Input: part model. Units: mm. Frame: model coordinates. A direction names the side the tool comes from. Round coordinates to 2 decimals unless told otherwise and drop trailing zeros. Write each loop counter-clockwise with the first axis right and the second up, starting at its lowest first coordinate (ties: lowest second). Pieces come first, ordered by that corner, then holes. Notation, with made-up numbers: (61.5, 57) - (79.5, 57) arc R30 ccw to (79.5, 89) - close; hole circle Ø8 at (-8, 26.5). An arc over 180 degrees is marked (long way). Use one line per item in the form item = value.
Autodesk Inventor part; units mm, degrees
ref_plane "Work Plane1" through (0, 0, -34) normal (0, 0, -1) x (-1, 0, 0)
ref_plane "Work Plane2" through (-19.4786, -19.4786, -43.1) normal (0, 0, -1) x (-0.6619, 0.7496, 0)
ref_plane "YZ Plane" through (0, 0, 0) normal (1, 0, 0) x (0, 1, 0)
ref_plane "Work Plane1" through (0, 0, -34) normal (0, 0, -1) x (-1, 0, 0)
sketch "Sketch1" plane through (0, 0, -34) normal (0, 0, -1) x (-1, 0, 0)
  line L0 (-15, 14.5) -> (-11.5, 14.5)
  line L1 (-15, 14.5) -> (-20.1, 8.5)
  line L2 (-20.1, 8.5) -> (-20.1, -44.6)
  line L3 (-20.1, -44.6) -> (-15, -50.6)
  line L4 (-15, -50.6) -> (15, -50.6)
  line L5 (15, -50.6) -> (20.1, -44.6)
  line L6 (20.1, -44.6) -> (20.1, 8.5)
  line L7 (20.1, 8.5) -> (15, 14.5)
  line L8 (11.5, 14.5) -> (15, 14.5)
  arc A0 (14.5, 11.5) -> (11.5, 14.5) centre (11.5, 11.5) ccw
  line L9 (14.5, -42) -> (14.5, 11.5)
  arc A1 (11.5, -45) -> (14.5, -42) centre (11.5, -42) ccw
  line L10 (-11.5, -45) -> (11.5, -45)
  arc A2 (-14.5, -42) -> (-11.5, -45) centre (-11.5, -42) ccw
  line L11 (-14.5, 11.5) -> (-14.5, -42)
  arc A3 (-11.5, 14.5) -> (-14.5, 11.5) centre (-11.5, 11.5) ccw
  circle A4 centre (17.3, 4) radius 1.35
  circle A5 centre (17.3, -18) radius 1.35
  circle A6 centre (17.3, -40) radius 1.35
  circle A7 centre (11, -47.8) radius 1.35
  circle A8 centre (-17.3, 4) radius 1.35
  circle A9 centre (-17.3, -18) radius 1.35
  circle A10 centre (-17.3, -40) radius 1.35
  circle A11 centre (-11, -47.8) radius 1.35
  line L12 (-20.1, -18.05) -> (-20.1, -15.05)
  line L13 (-20.1, -18.05) -> (-17.1, -18.05) construction
  line L14 (-20.1, -18.05) -> (-20.1, -44.6)
  line L15 (-20.1, -44.6) -> (-15, -50.6)
  line L16 (-15, -50.6) -> (15, -50.6)
  line L17 (15, -50.6) -> (20.1, -44.6)
  line L18 (20.1, -44.6) -> (20.1, -18.05)
  line L19 (20.1, -18.05) -> (20.1, -15.05)
  line L20 (20.1, -18.05) -> (23.1, -18.05) construction
  line L21 (20.1, -15.05) -> (-20.1, -15.05)
  point P0 (0, 0)
  dimension "d0" = 3
  dimension "d1" = 90
  dimension "d2" = 3
  dimension "d3" = 90
ref_plane "Work Plane2" through (-19.4786, -19.4786, -43.1) normal (0, 0, -1) x (-0.6619, 0.7496, 0)
extrude "Extrusion1" add sketch "Sketch1" along normal blind 10 contours L21 L11 A2 L10 A1 L9 L6 L5 L4 L3 L2 | L21 L9 A1 L10 A2 L11 | A7 | A11
sketch "Sketch2" plane through (0, 0, -34) normal (0, 0, 1) x (1, 0, 0)
  line L0 (15, 14.5) -> (11.5, 14.5)
  line L1 (15, 14.5) -> (20.1, 8.5)
  line L2 (20.1, 8.5) -> (20.1, -44.6)
  line L3 (20.1, -44.6) -> (15, -50.6)
  line L4 (15, -50.6) -> (-15, -50.6)
  line L5 (-15, -50.6) -> (-20.1, -44.6)
  line L6 (-20.1, -44.6) -> (-20.1, 8.5)
  line L7 (-20.1, 8.5) -> (-15, 14.5)
  line L8 (-11.5, 14.5) -> (-15, 14.5)
  arc A0 (-11.5, 14.5) -> (-14.5, 11.5) centre (-11.5, 11.5) ccw
  line L9 (-14.5, -42) -> (-14.5, 11.5)
  arc A1 (-14.5, -42) -> (-11.5, -45) centre (-11.5, -42) ccw
  line L10 (11.5, -45) -> (-11.5, -45)
  arc A2 (11.5, -45) -> (14.5, -42) centre (11.5, -42) ccw
  line L11 (14.5, 11.5) -> (14.5, -42)
  arc A3 (14.5, 11.5) -> (11.5, 14.5) centre (11.5, 11.5) ccw
  circle A4 centre (-17.3, 4) radius 1.35
  circle A5 centre (-17.3, -18) radius 1.35
  circle A6 centre (-17.3, -40) radius 1.35
  circle A7 centre (-11, -47.8) radius 1.35
  circle A8 centre (17.3, 4) radius 1.35
  circle A9 centre (17.3, -18) radius 1.35
  circle A10 centre (17.3, -40) radius 1.35
  circle A11 centre (11, -47.8) radius 1.35
  line L12 (-20.1, -15.05) -> (20.1, -15.05)
  line L13 (14.5, -15.05) -> (14.7, -15.05)
  line L14 (14.7, -15.05) -> (14.7, -40)
  line L15 (14.7, -15.05) -> (39.65, -15.05) construction
  line L16 (14.7, -40) -> (14.7, -43)
  line L17 (14.7, -43) -> (-14.7, -43)
  line L18 (-14.7, -43) -> (-14.7, -15.05)
  line L19 (-14.7, -15.05) -> (14.7, -15.05)
  line L20 (14.7, -15.05) -> (14.7, -43)
  point P0 (0, 0)
  dimension "d6" = 0.2
  dimension "d8" = 90
  dimension "d9" = 3
  dimension "d10" = 29.4
  dimension "d11" = 27.95
extrude "Extrusion2" cut sketch "Sketch2" against normal blind 6.3 contours L12 L14 L16 L17 A2 L11 | L11 A2 L17 A1 L9 L12 | L9 A1 L17 L18 L12
sketch "Sketch4" plane through (0, 0, -34) normal (0, 0, 1) x (1, 0, 0)
  line L0 (-14.7, -43) -> (-14.7, -15.05)
  line L1 (-14.7, -43) -> (-20.1, -43)
  line L2 (-20.1, -44.6) -> (-20.1, -15.05)
  line L3 (-20.1, -43) -> (20.1, -43)
  line L4 (20.1, -43) -> (20.1, -50.6)
  line L5 (20.1, -50.6) -> (-20.1, -50.6)
  line L6 (-20.1, -50.6) -> (-20.1, -43)
  point P0 (0, 0)
  dimension "d14" = 7.6
  dimension "d15" = 40.2
extrude "Extrusion3" cut sketch "Sketch4" against normal blind 6.3
sketch "Sketch5" plane through (0, 0, -44) normal (0, 0, -1) x (-1, 0, 0)
  line L0 (-20.1, -15.05) -> (-20.1, -44.6)
  line L1 (-20.1, -15.05) -> (-20.1, -36.05)
  line L2 (-20.1, -15.05) -> (0.9, -15.05) construction
  line L3 (-20.1, -36.05) -> (0, -36.05)
  line L4 (-20.1, -36.05) -> (0, -36.05) construction
  circle A0 centre (0, -36.05) radius 5.5
  line L5 (0, -36.05) -> (0, -47.05)
  line L6 (0, -36.05) -> (11, -36.05) construction
  circle A1 centre (0, -47.05) radius 1.025
  circle A2 centre (7.7782, -43.8282) radius 1.025
  circle A3 centre (11, -36.05) radius 1.025
  circle A4 centre (7.7782, -28.2718) radius 1.025
  circle A5 centre (0, -25.05) radius 1.025
  circle A6 centre (-7.7782, -28.2718) radius 1.025
  circle A7 centre (-11, -36.05) radius 1.025
  circle A8 centre (-7.7782, -43.8282) radius 1.025
  point P0 (0, 0)
  dimension "d18" = 21
  dimension "d19" = 90
  dimension "d23" = 20.1
  dimension "d24" = 0
  dimension "d25" = 11
  dimension "d26" = 11
  dimension "d27" = 90
  dimension "d28" = 2.05
  dimension "d31" = 360
extrude "Extrusion4" cut sketch "Sketch5" against normal up to surface (3.7 mm away)
sketch "Sketch7" plane through (0, 0, -44) normal (0, 0, -1) x (-1, 0, 0)
  circle A0 centre (-7.7782, -43.8282) radius 1.025 construction
  circle A1 centre (0, -36.05) radius 5.5 construction
  circle A2 centre (-11, -36.05) radius 1.025 construction
  circle A3 centre (0, -25.05) radius 1.025 construction
  circle A4 centre (11, -36.05) radius 1.025 construction
  circle A5 centre (0, -47.05) radius 1.025 construction
  circle A6 centre (7.7782, -43.8282) radius 1.025 construction
  circle A7 centre (7.7782, -28.2718) radius 1.025 construction
  circle A8 centre (-7.7782, -28.2718) radius 1.025 construction
  circle A9 centre (-17.3, -40) radius 1.35 construction
  circle A10 centre (-17.3, -18) radius 1.35 construction
  circle A11 centre (17.3, -40) radius 1.35 construction
  circle A12 centre (17.3, -18) radius 1.35 construction
  line L0 (-20.1, -44.6) -> (-15, -50.6) construction
  line L1 (-15, -50.6) -> (15, -50.6) construction
  line L2 (15, -50.6) -> (20.1, -44.6) construction
  line L3 (20.1, -44.6) -> (20.1, -15.05) construction
  line L4 (20.1, -15.05) -> (-20.1, -15.05) construction
  line L5 (-20.1, -15.05) -> (-20.1, -44.6) construction
  line L6 (-20.1, -15.05) -> (-20.1, -27.05)
  line L7 (-20.1, -15.05) -> (-20.1, -44.6) construction
  line L8 (-20.1, -15.05) -> (-8.1, -15.05)
  line L9 (0, -15.05) -> (0, -21.5) construction
  line L10 (0, -21.5) -> (20.1, -21.5) construction
  line L11 (0, -21.5) -> (20.1, -21.5) construction
  line L12 (0, -21.5) -> (-20.1, -21.5) construction
  line L13 (0, -21.5) -> (20.1, -21.5) construction
  line L14 (-20.1, -27.05) -> (-14.55, -21.5)
  line L15 (-20.1, -27.05) -> (-12.2511, -27.05) construction
  line L16 (0, -15.05) -> (20.1, -15.05)
  line L17 (20.1, -15.05) -> (20.1, -27.05)
  line L18 (20.1, -27.05) -> (14.55, -21.5)
  line L19 (14.55, -21.5) -> (-14.55, -21.5)
  line L20 (-14.7, -15.05) -> (-20.1, -15.05)
  line L21 (-20.1, -15.05) -> (20.1, -15.05)
  point P0 (0, 0)
  dimension "d40" = 12
  dimension "d41" = 90
  dimension "d42" = 6.45
  dimension "d43" = 20.1
  dimension "d44" = 0
  dimension "d45" = 20.1
  dimension "d46" = 180
  dimension "d47" = 45
  dimension "d48" = 12
  dimension "d49" = 90
  dimension "d50" = 45
extrude "Extrusion5" cut sketch "Sketch7" against normal blind 4
sketch "Sketch10" plane through (20.1, -44.6, -40.3) normal (1, 0, 0) x (0, 0, -1)
  line L0 (3.7, 17.55) -> (-0.3, 17.55) construction
  line L1 (-0.3, 17.55) -> (-0.3, 29.55) construction
  line L2 (-6.3, 29.55) -> (-0.3, 29.55) construction
  line L3 (-6.3, 29.55) -> (-6.3, 1.6) construction
  line L4 (-6.3, 1.6) -> (0, 1.6) construction
  line L5 (0, 1.6) -> (0, 0) construction
  line L6 (0, 0) -> (3.7, 0) construction
  line L7 (3.7, 17.55) -> (3.7, 0) construction
  line L8 (0, 0) -> (0, -6) construction
  line L9 (0, -6) -> (3.7, -6) construction
  line L10 (3.7, 0) -> (3.7, -6) construction
  line L11 (0, 0) -> (3.7, 0) construction
  line L12 (-6.3, 29.55) -> (-0.3, 29.55)
  line L13 (-6.3, 29.55) -> (3.7, 29.55)
  line L14 (3.7, 29.55) -> (3.7, -6)
  line L15 (3.7, -6) -> (-6.3, -6)
  line L16 (-6.3, -6) -> (-6.3, 29.55)
  point P0 (-40.3, 44.6)
sketch "Sketch12" plane through (-20.1, -44.6, -44) normal (-1, 0, 0) x (0, 0, 1)
  line L0 (4, 17.55) -> (0, 17.55) construction
  line L1 (0, 0) -> (0, 17.55) construction
  line L2 (3.7, 0) -> (0, 0) construction
  line L3 (3.7, 0) -> (3.7, 1.6) construction
  line L4 (3.7, 1.6) -> (10, 1.6) construction
  line L5 (10, 1.6) -> (10, 29.55) construction
  line L6 (10, 29.55) -> (4, 29.55) construction
  line L7 (4, 29.55) -> (4, 17.55) construction
  line L8 (3.7, -6) -> (3.7, 0) construction
  line L9 (3.7, 0) -> (0, 0) construction
  line L10 (0, -6) -> (0, 0) construction
  line L11 (3.7, -6) -> (0, -6) construction
  line L12 (10, 29.55) -> (4, 29.55)
  line L13 (3.7, -6) -> (0, -6)
  line L14 (10, 29.55) -> (0, 29.55)
  line L15 (0, 29.55) -> (0, -6)
  line L16 (0, -6) -> (10, -6)
  line L17 (10, -6) -> (10, 29.55)
  point P0 (44, 44.6)
extrude "Extrusion8" cut sketch "Sketch10" against normal blind 0.1
extrude "Extrusion9" cut sketch "Sketch12" against normal blind 0.1
fillet "Fillet2" radius 2 2 edges at (-20, -15.05, -37) (20, -15.05, -37)
properties part number "knee_connector_new"
(1) First-contact query: pin 1 Ø3 at (x, y) = (-17.3, -40) entering from -Z; pin 2 Ø3.5 at (x, y) = (-11, -36.05) entering from +Z; pin 3 Ø2 at (x, y) = (17.3, -40) entering from +Z; pin 4 Ø4 at (x, z) = (4, -41.5) entering from +Y. Flat tips, straight axial feed; report the tip coordinate or a pass-through.
Derived:
pin_1 = -44
pin_2 = -40.3
pin_3 = through
pin_4 = -21.5
(2) Cut plane D-D on y = -23. Output: boundary loops of the cut face in (x, z).
Derived:
outline = (-20, -40) - (-16.05, -40) - (-16.05, -44) - (16.05, -44) - (16.05, -40) - (20, -40) - (20, -34) - (14.7, -34) - (14.7, -40.3) - (-14.7, -40.3) - (-14.7, -34) - (-20, -34) - close
(3) Cut plane A-A on x = 0. Output: boundary loops of the cut face in (y, z) (3 decimals), then the cut area to 3 significant figures.
Derived:
outline = (-50.6, -44) - (-48.075, -44) - (-48.075, -40.3) - (-50.6, -40.3) - close; (-46.025, -44) - (-41.55, -44) - (-41.55, -40.3) - (-46.025, -40.3) - close; (-30.55, -44) - (-26.075, -44) - (-26.075, -40.3) - (-30.55, -40.3) - close; (-24.025, -44) - (-21.5, -44) - (-21.5, -40.3) - (-24.025, -40.3) - close
area = 51.8 mm^2
(4) Cut plane C-C on x = -11. Output: boundary loops of the cut face in (y, z) (3 decimals), then the cut area to 3 significant figures.
Derived:
outline = (-50.6, -44) - (-37.075, -44) - (-37.075, -40.3) - (-50.6, -40.3) - close; (-35.025, -44) - (-21.5, -44) - (-21.5, -40.3) - (-35.025, -40.3) - close
area = 100 mm^2
(5) Draft query along X for faces 4 (the face through (-14.7, -29, -37)), 5 (the face through (-17.465, -47.7, -42.124)), 6 (the face through (-17, -20, -40)). Return one class per face: released by +X, released by -X, zero draft, split by the parting line, or undercut.
Derived:
face_4 = undercut
face_5 = released by -X
face_6 = zero draft
(6) Cut plane B-B on z = -37.5. Output: boundary loops of the cut face in (x, y).
Derived:
outline = (-20, -43) - (-14.7, -43) - (-14.7, -15.05) - (-18, -15.05) arc R2 ccw to (-20, -17.05) - close; (14.7, -43) - (20, -43) - (20, -17.05) arc R2 ccw to (18, -15.05) - (14.7, -15.05) - close; hole circle Ø2.7 at (-17.3, -40); hole circle Ø2.7 at (-17.3, -18); hole circle Ø2.7 at (17.3, -40); hole circle Ø2.7 at (17.3, -18)
(7) Material intervals for L1, parallel to Y at x = 0, z = -42 (3 decimals); L2, parallel to Y at x = 17.3, z = -36.75; L3, parallel to X at y = -18, z = -35.8, sorted ascending.
Derived:
L1 = -50.6 to -48.075, -46.025 to -41.55, -30.55 to -26.075, -24.025 to -21.5
L2 = -43 to -41.35, -38.65 to -19.35, -16.65 to -15.05
L3 = -20 to -18.65, -15.95 to -14.7, 14.7 to 15.95, 18.65 to 20
(8) Access query for faces 1 (the face through (17.31, -24.26, -42.03)), 2 (the face through (-17.31, -24.26, -42.03)), 3 (the face through (14.7, -29, -37)). Directions: +Z, -Z, +X, -X, +Y, -Y. A direction counts if a zero-diameter tool reaches every point of the face in a straight line with its end or side. Return the directions, or none.
Derived:
face_1 = -Z, +X, +Y
face_2 = -Z, -X, +Y
face_3 = +Z, +Y, -Y
